The listing builds one solid part. Answer for the finished solid, in the listing's coordinates (mm). Give positions to 0.01 mm unless a question says otherwise; leave off trailing zeros. Write each loop counter-clockwise with the first axis right and the second up, starting at its lowest first coordinate (ties: lowest second). Pieces come first, ordered by that corner, then holes.
```python
from build123d import *

# Parameters (mm, degrees)
SKETCH_1_W          = 140
SKETCH_1_H          = 60
EXTRUDE_1_DEPTH     = 1.6
SKETCH_2_R          = 1.5
CUT_EXTRUDE_1_DEPTH = 1.6
SKETCH_3_R          = 1.5
CUT_EXTRUDE_2_DEPTH = 1.6


with BuildPart() as part:
    # Эскиз1 → Бобышка-Вытянуть1 (new body)
    with BuildSketch(Plane(origin=(0, 0, 0), x_dir=(1, 0, 0), z_dir=(0, 1, 0))):
        Rectangle(SKETCH_1_W, SKETCH_1_H)
    extrude(amount=EXTRUDE_1_DEPTH)

    # Эскиз2 → Вырез-Вытянуть1 (cut)
    with BuildSketch(Plane(origin=(0, 1.6, 0), x_dir=(1, 0, 0), z_dir=(0, 1, 0))):
        with Locations(Location((-66, 26, 0), (0, 0, 270))):
            Circle(SKETCH_2_R)
        with Locations(Location((-66, -26, 0), (0, 0, 270))):
            Circle(SKETCH_2_R)
        with Locations(Location((66, -26, 0), (0, 0, 270))):
            Circle(SKETCH_2_R)
        with Locations(Location((66, 26, 0), (0, 0, 270))):
            Circle(SKETCH_2_R)
    extrude(amount=-CUT_EXTRUDE_1_DEPTH, mode=Mode.SUBTRACT)

    # Эскиз3 → Вырез-Вытянуть2 (cut)
    with BuildSketch(Plane(origin=(0, 1.6, 0), x_dir=(1, 0, 0), z_dir=(0, 1, 0))):
        with Locations(Location((-52.5, 27.5, 0), (0, 0, 270))):
            Circle(SKETCH_3_R)
        with Locations(Location((-52.5, -27.5, 0), (0, 0, 270))):
            Circle(SKETCH_3_R)
        with Locations(Location((40.5, 27.5, 0), (0, 0, 270))):
            Circle(SKETCH_3_R)
        with Locations(Location((40.5, -27.5, 0), (0, 0, 270))):
            Circle(SKETCH_3_R)
    extrude(amount=-CUT_EXTRUDE_2_DEPTH, mode=Mode.SUBTRACT)


solid = part.part
```
Item 1: Each of these flat-tipped pins is pushed along its axis until it touches: P1, Ø2, axis at x = -16, z = 17, coming from the -Y side; P2, Ø1.8, axis at x = -52.5, z = 27.5, coming from the +Y side (3 decimals). Where does it stop, or does it pass through?
Conclusion:
P1: stops at y = 0
P2: passes through
Item 2: A cutting plane is placed at A-A, the plane x = 66. Give the vertices of the cut face in (y, z), plus the area to 3 significant figures.
Conclusion:
outline: (0, -30) - (1.6, -30) - (1.6, -27.5) - (0, -27.5) - close; (0, -24.5) - (1.6, -24.5) - (1.6, 24.5) - (0, 24.5) - close; (0, 27.5) - (1.6, 27.5) - (1.6, 30) - (0, 30) - close
area: 86.4 mm2
Item 3: Determine the mould class of faces 1 (the face through (-1, 0, 0)), 2 (the face through (39.6, 0.8, -28.7)) for opening direction X: pulls with the +X half, pulls with the -X half, needs draft (parallel to the pull), parting line crosses it, or undercut.
Conclusion:
face 1: needs draft
face 2: undercut
